Input: part model. Units: mm. Frame: model coordinates. Face numbers are marked on the shaded views. Round coordinates to 2 decimals unless told otherwise and drop trailing zeros. Loops run counter-clockwise (first coordinate to the right, second up) from the corner with the lowest first, then second, coordinate; pieces in that order, holes last. Notation, with made-up numbers: (24, 72) -> (79, 72) arc R13 ccw to (79, 97) -> close; hole circle Ø2 at (-32, 9.5). An arc over 180 degrees is marked (long way). Answer as a JSON object with one key per item and string values.
```python
from build123d import *

# Parameters (mm, degrees)
SKETCH12_R                    = 161.925
SKETCH12_R_2                  = 152.4
PIPE_STANDARD_S40_P12_2_DEPTH = 508
SKETCH13_R                    = 3.175
CUT_EXTRUDE1_DEPTH            = 558.228329547
SKETCH15_R                    = 3.175
CUT_EXTRUDE2_DEPTH            = 558.228329706
SKETCH16_R                    = 3.175
CUT_EXTRUDE3_DEPTH            = 558.228329706


with BuildPart() as part:
    # Sketch12 → Pipe (standard, s40) P12(2) (new body)
    with BuildSketch(Plane.XZ):
        Circle(SKETCH12_R)
        Circle(SKETCH12_R_2, mode=Mode.SUBTRACT)
    extrude(amount=PIPE_STANDARD_S40_P12_2_DEPTH)

    # Sketch13 → Cut-Extrude1 (cut, through all)
    with BuildSketch(Plane.XY):
        with Locations(Location((0, -482.6, 0), (0, 0, 180))):
            Circle(SKETCH13_R)
        with Locations(Location((0, -25.4, 0), (0, 0, 180))):
            Circle(SKETCH13_R)
    extrude(amount=CUT_EXTRUDE1_DEPTH, mode=Mode.SUBTRACT)

    # Sketch15 → Cut-Extrude2 (cut, through all)
    with BuildSketch(Plane(origin=(0, 0, 0), x_dir=(0, -1, 0), z_dir=(-0.7071067811865438, 0, -0.7071067811865512))):
        with Locations(Location((482.6, 0, 0), (0, 0, 90))):
            Circle(SKETCH15_R)
    extrude(amount=-CUT_EXTRUDE2_DEPTH, mode=Mode.SUBTRACT)

    # Sketch16 → Cut-Extrude3 (cut, through all)
    with BuildSketch(Plane(origin=(0, 0, 0), x_dir=(0, 0, -1), z_dir=(1, 0, 0))):
        with Locations(Location((0, -482.6, 0), (0, 0, 90.000000043))):
            Circle(SKETCH16_R)
    extrude(amount=CUT_EXTRUDE3_DEPTH, mode=Mode.SUBTRACT)


solid = part.part
```
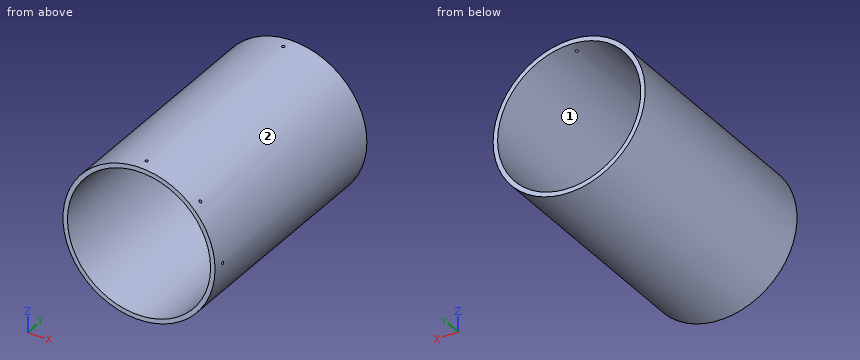
1) Section A-A, the plane x = 27. Output: boundary loops of the cut face in (y, z), plus the area to 3 significant figures.
Output:
{"outline": "(-508, -159.66) -> (0, -159.66) -> (0, -149.99) -> (-508, -149.99) -> close; (-508, 149.99) -> (0, 149.99) -> (0, 159.66) -> (-508, 159.66) -> close", "area": "9,820 mm^2"}
2) Section C-C, the plane y = -306.5. Output: boundary loops of the cut face in (x, z) (3 decimals).
Output:
{"outline": "circle Ø323.85 at (0, 0); hole circle Ø304.8 at (0, 0)"}
3) Ray query, probe 1 along X at (y, z) = (-115, -1.5); probe 2 along Z at (x, y) = (0, -352) (3 decimals); probe 3 along Z at (x, y) = (-38, -456). Return the intervals inside material, ascending.
Output:
{"probe 1": "x = -161.92 to -152.39, 152.39 to 161.92", "probe 2": "z = -161.925 to -152.4, 152.4 to 161.925", "probe 3": "z = -157.4 to -147.59, 147.59 to 157.4"}
4) Section B-B, the plane z = -112. Output: boundary loops of the cut face in (x, y), plus the area to 3 significant figures.
Output:
{"outline": "(-116.94, -508) -> (-103.35, -508) -> (-103.35, 0) -> (-116.94, 0) -> close; (103.35, -508) -> (116.94, -508) -> (116.94, 0) -> (103.35, 0) -> close", "area": "13,800 mm^2"}
5) Contact query for flat-ended pins moving along their axis: P1, Ø10, axis at x = -112.5, y = -394.5, coming from the +Z side; P2, Ø3, axis at y = -269, z = 101, coming from the +X side; P3, Ø2, axis at y = -149, z = 100.5, coming from the -X side. Output: stop coordinate, or through.
Output:
{"P1": "stops at z = 121.09", "P2": "stops at x = 127.75", "P3": "stops at x = -127.75"}
6) Draft query along X for the marked faces 1 and 2. Return one class per face: +X half, -X half, draft (parallel to the pull), parting line (faces both ways), or undercut.
Output:
{"face 1": "undercut", "face 2": "parting line"}
